from build123d import *

# Parameters (mm, degrees)
SKETCH1_W           = 100
SKETCH1_H           = 100
BOSS_EXTRUDE1_DEPTH = 800
SKETCH2_W           = 100
SKETCH2_H           = 100
BOSS_EXTRUDE2_DEPTH = 700
BOSS_EXTRUDE3_DEPTH = 100
SKETCH5_R           = 25
BOSS_EXTRUDE4_DEPTH = 25
CUT_EXTRUDE2_DEPTH  = 801
BOSS_EXTRUDE5_DEPTH = 100
CUT_EXTRUDE3_DEPTH  = 801
SKETCH10_R          = 25
BOSS_EXTRUDE6_DEPTH = 30


with BuildPart() as part:
    # Sketch1 → Boss-Extrude1 (new body)
    with BuildSketch(Plane.XY):
        with Locations((50, 50)):
            Rectangle(SKETCH1_W, SKETCH1_H)
    extrude(amount=BOSS_EXTRUDE1_DEPTH)

    # Sketch2 → Boss-Extrude2 (add)
    with BuildSketch(Plane(origin=(0, 0, 0), x_dir=(0, 0, -1), z_dir=(1, 0, 0))):
        with Locations((-750, 50)):
            Rectangle(SKETCH2_W, SKETCH2_H)
    extrude(amount=-BOSS_EXTRUDE2_DEPTH)

    # Sketch4 → Boss-Extrude3 (add)
    with BuildSketch(Plane.XY.offset(800)):
        Polygon((-493.990986432, 0), (-600, -41.564522078), (-600, -730.356100977), (-700, -730.356100977), (-700, 0), align=None)
    extrude(amount=-BOSS_EXTRUDE3_DEPTH)

    # Sketch5 → Boss-Extrude4 (add)
    with BuildSketch(Plane(origin=(0, -730.356100977, 0), x_dir=(-1, 0, 0), z_dir=(0, -1, 0))):
        with Locations((650, -750)):
            Circle(SKETCH5_R)
    extrude(amount=BOSS_EXTRUDE4_DEPTH)

    # Sketch6 → Cut-Extrude2 (cut, through all)
    with BuildSketch(Plane.XY.offset(800)):
        Polygon((-700, 0), (-700, 77.872935738), (-481.374152596, 0), align=None)
    extrude(amount=-CUT_EXTRUDE2_DEPTH, mode=Mode.SUBTRACT)

    # Sketch8 → Boss-Extrude5 (add)
    with BuildSketch(Plane.XY.offset(800)):
        Polygon((-700, 100), (-600, 100), (-481.374152596, 100), (-600, 139.764231535), (-600, 826.035666916), (-700, 826.035666916), align=None)
    extrude(amount=-BOSS_EXTRUDE5_DEPTH)

    # Sketch9 → Cut-Extrude3 (cut, through all)
    with BuildSketch(Plane.XY.offset(800)):
        Polygon((-740.353325761, 0), (-493.364641431, 0), (-493.364641431, -882.481689371), (-837.990616097, -863.88243179), align=None)
    extrude(amount=-CUT_EXTRUDE3_DEPTH, mode=Mode.SUBTRACT)

    # Sketch10 → Boss-Extrude6 (add)
    with BuildSketch(Plane(origin=(0, 826.035666916, 0), x_dir=(1, 0, 0), z_dir=(0, 1, 0))):
        with Locations((-650, -750)):
            Circle(SKETCH10_R)
    extrude(amount=BOSS_EXTRUDE6_DEPTH)


solid = part.part
Model file for the job. Use its own axes, mm. A direction names the side the tool comes from. Round coordinates to 2 decimals unless told otherwise and drop trailing zeros. Order: outer loops, then holes, each group sorted by start corner. A loop starts at its lowest first (then second) coordinate and runs counter-clockwise, first axis right, second up.
(1) Drill centre lines: line 1 (Y direction, x = 1, z = 749.5); line 2 (X direction, y = 368, z = 767). Where is each one in solid material? Low to high.
(2) Band-saw the part on A-A (z = 750). List the corners of the cut face in (x, y).
(3) Band-saw the part on C-C (y = 320). List the corners of the cut face in (x, z), then the cut area to 3 significant figures.
(4) Band-saw the part on D-D (x = -650). List the corners of the cut face in (y, z), then the cut area to 3 significant figures.
(5) Pin check, flat tip, straight feed: pin 1 (6 mm diameter, centred on x = -419.5, y = 102, fed in from -Z). Stop position of the tip, or through.
(6) Band-saw the part on B-B (x = -327.5). List the corners of the cut face in (y, z).
(7) 3-axis set-ups, long thin cutter, end or side, ignore diameter. For faces 1 (the face through (-638.5, 840.8, 772.2)), 2 (the face through (0, 49, 345)), 3 (the face through (-600, 478, 751)): which of +Z, -Z, +X, -X, +Y, -Y reach the whole face in a straight line?
Verdict:
1. line 1: y = 0 to 100
1. line 2: x = -700 to -600
2. outline: (-700, 77.87) - (-481.37, 0) - (100, 0) - (100, 100) - (-481.37, 100) - (-600, 139.76) - (-600, 826.04) - (-625, 826.04) - (-625, 856.04) - (-675, 856.04) - (-675, 826.04) - (-700, 826.04) - close
3. outline: (-700, 700) - (-600, 700) - (-600, 800) - (-700, 800) - close
3. area: 10,000 mm2
4. outline: (60.06, 700) - (826.04, 700) - (826.04, 725) - (856.04, 725) - (856.04, 775) - (826.04, 775) - (826.04, 800) - (60.06, 800) - close
4. area: 78,100 mm2
5. pin 1: stops at z = 700
6. outline: (0, 700) - (100, 700) - (100, 800) - (0, 800) - close
7. face 1: +Y
7. face 2: -Z, -X, +Y, -Y
7. face 3: +Z, -Z, +X, +Y
